Read the model definition and answer for the solid it produces. Units are mm, in the model's axes. A direction names the side the tool comes from. Round coordinates to 2 decimals unless told otherwise and drop trailing zeros. Order: outer loops, then holes, each group sorted by start corner. A loop starts at its lowest first (then second) coordinate and runs counter-clockwise, first axis right, second up. Notation, with made-up numbers: (68.5, 8.5) - (113.5, 8.5) arc R22 cw to (113.5, 22.5) - close; hole circle Ø3 at (0.25, -22.5). An arc over 180 degrees is marked (long way). Answer as a JSON object with one key per item and string values. Group by question number.
Q1. Given pin 1 Ø7 at (x, y) = (66.5, 6) entering from +Z; pin 2 Ø4 at (x, y) = (7, 32.5) entering from -Z, each flat-ended and moving along its own axis, determine where each tip first touches the part or whether it passes through.
Q2. A cutting plane is placed at D-D on x = 34.5. Determine the outline of the cut face in (y, z), and give its area (3 significant figures).
Q3. A tool of negligible diameter and unlimited length cuts with its end or side. For faces 1 (the cylindrical face through (22.534, 6.521, 12.566)), 2 (the cylindrical face through (71.93, 39.4, 7.6)), from which of +Z, -Z, +X, -X, +Y, -Y can it reach the whole face along a straight path? Write none if from no direction.
Q4. A cutting plane is placed at C-C on z = 13.25. Determine the outline of the cut face in (x, y).
Q5. A cutting plane is placed at A-A on x = 7. Determine the outline of the cut face in (y, z), and give its area (3 significant figures).
Q6. A cutting plane is placed at B-B on y = 11.5. Determine the outline of the cut face in (x, z), and give its area (3 significant figures).
Q7. The mould has two halves that part along Y. Classify faces 3 (the cylindrical face through (0.6, 39.43, 7.6)), 4 (the cylindrical face through (70.405, 6.867, 12.566)), 5 (the cylindrical face through (0.57, 0.6, 7.6)), 6 (the cylindrical face through (23.8, 36.95, 12.57)): pulls with the +Y half, pulls with the -Y half, needs draft (parallel to the pull), parting line crosses it, or undercut.
Q8. Consider line 1 (Y direction, x = 66.5, z = 3.75); line 2 (Y direction, x = 38, z = 9.5); line 3 (X direction, y = 34, z = 11.25). Determine where each line is inside the solid, lowest interval first.
Solid Edge part; units mm, degrees
sketch "Sketch1" plane through (0, 0, 0) normal (0, 0, 1) x (1, 0, 0)
  line L0 (72.5, 40) -> (0, 40)
  line L1 (0, 40) -> (0, 0)
  line L2 (0, 0) -> (72.5, 0)
  line L3 (72.5, 0) -> (72.5, 40)
extrude "Extrusionsausprägung_1" add sketch "Sketch1" along normal blind 15
hole "Bohrung_1" at (26.5, 34, 15) direction (0, 0, -1) diameter 4.5 end through all counterbore diameter 8 counterbore depth 4.8
hole "Hole1" at (26.5, 6, 15) direction (0, 0, -1) diameter 4.5 end through all counterbore diameter 8 counterbore depth 4.8
hole "Hole2" at (66.5, 34, 15) direction (0, 0, -1) diameter 4.5 end through all counterbore diameter 8 counterbore depth 4.8
hole "Hole3" at (66.5, 6, 15) direction (0, 0, -1) diameter 4.5 end through all counterbore diameter 8 counterbore depth 4.8
hole "Bohrung_12" at (37.5, 20, 15) direction (0, 0, -1) diameter 20 end through all
hole "Bohrung_15" at (7, 32.5, 15) direction (0, 0, -1) diameter 6.5 end through all
hole "Hole4" at (7, 7.5, 15) direction (0, 0, -1) diameter 6.5 end through all
fillet "Verrundung_2" radius 2 4 edges at (0, 40, 7.5) (72.5, 40, 7.5) (72.5, 0, 7.5) (0, 0, 7.5)
Result set:
{
 "1": {"pin 1": "stops at z = 10.2", "pin 2": "passes through"},
 "2": {"outline": "(0, 0) - (10.46, 0) - (10.46, 15) - (0, 15) - close; (29.54, 0) - (40, 0) - (40, 15) - (29.54, 15) - close", "area": "314 mm²"},
 "3": {"face 1": "+Z", "face 2": "+Z, -Z, +X, +Y"},
 "4": {"outline": "(0, 2) arc R2 ccw to (2, 0) - (70.5, 0) arc R2 ccw to (72.5, 2) - (72.5, 38) arc R2 ccw to (70.5, 40) - (2, 40) arc R2 ccw to (0, 38) - close; hole circle Ø6.5 at (7, 7.5); hole circle Ø6.5 at (7, 32.5); hole circle Ø8 at (26.5, 6); hole circle Ø8 at (26.5, 34); hole circle Ø20 at (37.5, 20); hole circle Ø8 at (66.5, 6); hole circle Ø8 at (66.5, 34)"},
 "5": {"outline": "(0, 0) - (4.25, 0) - (4.25, 15) - (0, 15) - close; (10.75, 0) - (29.25, 0) - (29.25, 15) - (10.75, 15) - close; (35.75, 0) - (40, 0) - (40, 15) - (35.75, 15) - close", "area": "405 mm²"},
 "6": {"outline": "(0, 0) - (32.23, 0) - (32.23, 15) - (0, 15) - close; (42.77, 0) - (72.5, 0) - (72.5, 15) - (42.77, 15) - close", "area": "929 mm²"},
 "7": {"face 3": "pulls with the +Y half", "face 4": "undercut", "face 5": "pulls with the -Y half", "face 6": "undercut"},
 "8": {"line 1": "y = 0 to 3.75, 8.25 to 31.75, 36.25 to 40", "line 2": "y = 0 to 10.01, 29.99 to 40", "line 3": "x = 0 to 4.12, 9.88 to 22.5, 30.5 to 62.5, 70.5 to 72.5"}
}
